```python
from build123d import *

# Parameters (mm, degrees)
F1_DEPTH = 5.2
F2_R     = 10
F3_DEPTH = 4
F4_R     = 0.35
F5_DEPTH = 4


with BuildPart() as f1:
    # F0 (on Top) → F1 (new body)
    with BuildSketch(Plane.XY):
        with BuildLine():
            Line((7.496499, 8.05), (-7.496499, 8.05))
            ThreePointArc((-7.496499, 8.05), (-9.061942, 6.235479), (-10.197273, 4.125))
            ThreePointArc((-10.197273, 4.125), (-10.565281, 3.670844), (-11.124298, 3.5))
            Line((-11.124298, 3.5), (-14.25, 3.5))
            Line((-14.25, 3.5), (-14.25, -3.5))
            Line((-14.25, -3.5), (-11.124298, -3.5))
            ThreePointArc((-11.124298, -3.5), (-10.565281, -3.670844), (-10.197273, -4.125))
            ThreePointArc((-10.197273, -4.125), (-9.061942, -6.235479), (-7.496499, -8.05))
            Line((-7.496499, -8.05), (7.496499, -8.05))
            ThreePointArc((7.496499, -8.05), (9.061942, -6.235479), (10.197273, -4.125))
            ThreePointArc((10.197273, -4.125), (10.565281, -3.670844), (11.124298, -3.5))
            Line((11.124298, -3.5), (14.25, -3.5))
            Line((14.25, -3.5), (14.25, 3.5))
            Line((14.25, 3.5), (11.124298, 3.5))
            ThreePointArc((11.124298, 3.5), (10.565281, 3.670844), (10.197273, 4.125))
            ThreePointArc((10.197273, 4.125), (9.061942, 6.235479), (7.496499, 8.05))
        make_face()
    extrude(amount=F1_DEPTH)

    # F2 (on face) → F3 (cut)
    with BuildSketch(Plane(origin=(0, 0, 0), x_dir=(1, 0, 0), z_dir=(0, 0, -1))):
        Circle(F2_R)
    extrude(amount=-F3_DEPTH, mode=Mode.SUBTRACT)

    # F4 (on face) → F5 (join)
    with BuildSketch(Plane.XY.offset(5.2)):
        with Locations((13.45, 0)):
            Circle(F4_R)
        with Locations((-13.45, 1.27)):
            Circle(F4_R)
        with Locations((-13.45, -1.27)):
            Circle(F4_R)
    extrude(amount=F5_DEPTH)


solid = f1.part
```
Build history of the part. All positions in model axes, mm. A direction names the side the tool comes from. Round coordinates to 2 decimals unless told otherwise and drop trailing zeros. Order: outer loops, then holes, each group sorted by start corner. A loop starts at its lowest first (then second) coordinate and runs counter-clockwise, first axis right, second up. Notation, with made-up numbers: (75.25, -27) -> (84.25, -27) arc R11 cw to (84.25, -13) -> close; hole circle Ø10 at (-25.75, 78.5). An arc over 180 degrees is marked (long way). Answer in a Markdown table with one row per item.
1) Which spindle directions (+Z, -Z, +X, -X, +Y, -Y) get a long thin tool onto all of the face, cutting with end or side? Do faces 5 (the flat face through (-0.1, -8.05, 4.3)), 6 (the flat face through (-13, 3.5, 3)), 7 (the flat face through (13, 3.5, 3)), 8 (the flat face through (13, -3.5, 3)), 9 (the cylindrical face through (10, 0, 2)). Say none if no direction does.
Values:
| item | result |
|---|---|
| face 5 | +Z, -Z, +X, -X, -Y |
| face 6 | +Z, -Z, -X, +Y |
| face 7 | +Z, -Z, +X, +Y |
| face 8 | +Z, -Z, +X, -Y |
| face 9 | -Z |
2) Band-saw the part on B-B on x = -13.45. Give the cut face in (y, z), and give its area (3 significant figures).
Values:
| item | result |
|---|---|
| outline | (-3.5, 0) -> (3.5, 0) -> (3.5, 5.2) -> (1.62, 5.2) -> (1.62, 9.2) -> (0.92, 9.2) -> (0.92, 5.2) -> (-0.92, 5.2) -> (-0.92, 9.2) -> (-1.62, 9.2) -> (-1.62, 5.2) -> (-3.5, 5.2) -> close |
| area | 42.0 mm2 |
3) Mould opens along X. For faces 1 (the flat face through (0, 0, 4)), 2 (the flat face through (-14.25, 0, 3)), 3 (the cylindrical face through (-10, 0, 2)), 4 (the flat face through (-13, -3.5, 3)) say: released by +X, released by -X, zero draft, split by the parting line, or undercut.
Values:
| item | result |
|---|---|
| face 1 | undercut |
| face 2 | released by -X |
| face 3 | undercut |
| face 4 | zero draft |
4) Pin check, flat tips, straight feed: P1, Ø0.9, axis at x = -12.5, z = 1.5, coming from the -Y side; P2, Ø8, axis at x = 1, y = -3, coming from the -Z side; P3, Ø0.9, axis at x = -13, z = 3, coming from the +Y side; P4, Ø1, axis at x = -8, z = 6.5, coming from the +Y side. Stop position of each tip, or through.
Values:
| item | result |
|---|---|
| P1 | y = -3.5 |
| P2 | z = 4 |
| P3 | y = 3.5 |
| P4 | through |
5) Band-saw the part on C-C on y = 0. Give the cut face in (x, z).
Values:
| item | result |
|---|---|
| outline | (-14.25, 0) -> (-10, 0) -> (-10, 4) -> (10, 4) -> (10, 0) -> (14.25, 0) -> (14.25, 5.2) -> (13.8, 5.2) -> (13.8, 9.2) -> (13.1, 9.2) -> (13.1, 5.2) -> (-14.25, 5.2) -> close |
6) Wall check: L1, parallel to X at y = -0.25, z = 2.5; L2, parallel to Z at x = 10.75, y = -2.5; L3, parallel to Z at x = 4.25, y = -5.5. Give the ranges that are in metal, low to high.
Values:
| item | result |
|---|---|
| L1 | -14.25 to -10, 10 to 14.25 |
| L2 | 0 to 5.2 |
| L3 | 4 to 5.2 |
7) Band-saw the part on D-D on z = 6. Give the cut face in (x, y), and give its area (3 significant figures).
Values:
| item | result |
|---|---|
| outline | circle Ø0.7 at (-13.45, -1.27); circle Ø0.7 at (-13.45, 1.27); circle Ø0.7 at (13.45, 0) |
| area | 1.15 mm2 |
